The model under review builds one solid part; all positions refer to its coordinate system, in mm. Face numbers are marked on the shaded views. A direction names the side the tool comes from. Round coordinates to 2 decimals unless told otherwise and drop trailing zeros. Order: outer loops, then holes, each group sorted by start corner. A loop starts at its lowest first (then second) coordinate and runs counter-clockwise, first axis right, second up. Notation, with made-up numbers: M 53.5,39.5 L 101.5,39.5 A6 ccw 101.5,50.5 Z; hole C -34,18 d10. An arc over 180 degrees is marked long. Answer as a JSON object with one key per item and string values. Group by question number.
1. Add section C-C on x = 19.5. State the section outline as (y, z) points.
2. Add section A-A on y = 24. State the section outline as (x, z) points.
3. Add section B-B on z = 11. State the section outline as (x, y) points.
4. To check wall thickness, follow probe 1 along Y at (x, z) = (43.5, 11.25); probe 2 along X at (y, z) = (46.5, 16.5). State the ranges of each line that lie inside material, in increasing order. Write a range as [from, to].
5. Machinability: for the marked faces 1 and 2, which of the approach directions +Z, -Z, +X, -X, +Y, -Y give a long, thin tool a straight path to every point of the face, cutting with its end or side? Answer none if there is none.
6. Clearance check with flat-ended pins moving along their axes: P1, Ø12, axis at y = 44.5, z = 15, coming from the +X side; P2, Ø7.5, axis at x = 35.5, z = 9.5, coming from the +Y side. State where each tip first meets the part, or that it passes through.
```python
from build123d import *

# Parameters (mm, degrees)
SKETCH1_W           = 50
SKETCH1_H           = 18.5
BOSS_EXTRUDE1_DEPTH = 25
SKETCH2_W           = 15.5
SKETCH2_H           = 25
BOSS_EXTRUDE2_DEPTH = 50


with BuildPart() as part:
    # Sketch1 → Boss-Extrude1 (new body)
    with BuildSketch(Plane.XY):
        with Locations((25, 9.25)):
            Rectangle(SKETCH1_W, SKETCH1_H)
    extrude(amount=BOSS_EXTRUDE1_DEPTH)

    # Sketch2 → Boss-Extrude2 (add)
    with BuildSketch(Plane.XZ):
        with Locations((7.75, 12.5)):
            Rectangle(SKETCH2_W, SKETCH2_H)
    extrude(amount=-BOSS_EXTRUDE2_DEPTH)


solid = part.part
```
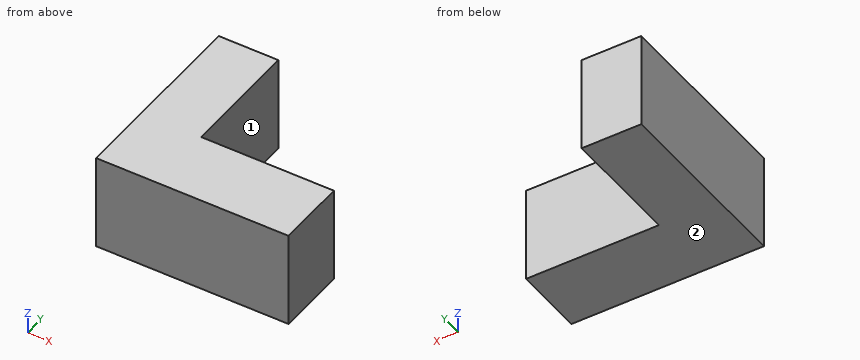
Recorded:
{
 "1": {"outline": "M 0,0 L 18.5,0 L 18.5,25 L 0,25 Z"},
 "2": {"outline": "M 0,0 L 15.5,0 L 15.5,25 L 0,25 Z"},
 "3": {"outline": "M 0,0 L 50,0 L 50,18.5 L 15.5,18.5 L 15.5,50 L 0,50 Z"},
 "4": {"probe 1": "y = [0, 18.5]", "probe 2": "x = [0, 15.5]"},
 "5": {"face 1": "+Z, -Z, +X, +Y", "face 2": "-Z, +X, -X, +Y, -Y"},
 "6": {"P1": "stops at x = 15.5", "P2": "stops at y = 18.5"}
}
